Geometry check sheet. Reference: the model listing, model coordinates, mm. Face numbers are marked on the shaded views. A direction names the side the tool comes from. Round coordinates to 2 decimals unless told otherwise and drop trailing zeros. Order: outer loops, then holes, each group sorted by start corner. A loop starts at its lowest first (then second) coordinate and runs counter-clockwise, first axis right, second up.
(1) Sectioned sample at B-B (x = -46.05). Record the boundary of the cut face in (y, z), plus the area to 4 significant figures.
(2) Go/stop test with flat-tipped pins: pin 1 (7.5 mm diameter, centred on y = 10.5, z = -4.5, fed in from +X); pin 2 (15.5 mm diameter, centred on x = -6.5, z = 2.5, fed in from +Y); pin 3 (1 mm diameter, centred on x = 2, z = -17.5, fed in from -Y). Record where each tip stops, or that it passes through.
(3) Release check for a two-part mould opening along Z. For the marked faces 4, 5 and 6 record: +Z half, -Z half, draft (parallel to the pull), parting line (faces both ways), or undercut.
(4) Sectioned sample at C-C (z = 0). Give the number of separate pieces and of enclosed holes in the cut face, plus the area to 3 significant figures.
(5) Sectioned sample at A-A (y = 13.5). Record the boundary of the cut face in (x, z).
(6) Sectioned sample at D-D (x = -28.5). Record the boundary of the cut face in (y, z), plus the area to 3 significant figures.
(7) Set-up check for the marked faces 1, 2 and 3: record each of +Z, -Z, +X, -X, +Y, -Y from which the full face is reachable in a straight line by a thin tool's end or side.
(8) Material ranges on line 1 along Y through (x, z) = (7, 15); line 2 along X through (y, z) = (1.8, 20.9); line 3 along Z through (x, y) = (16, 1.5), recorded low to high.
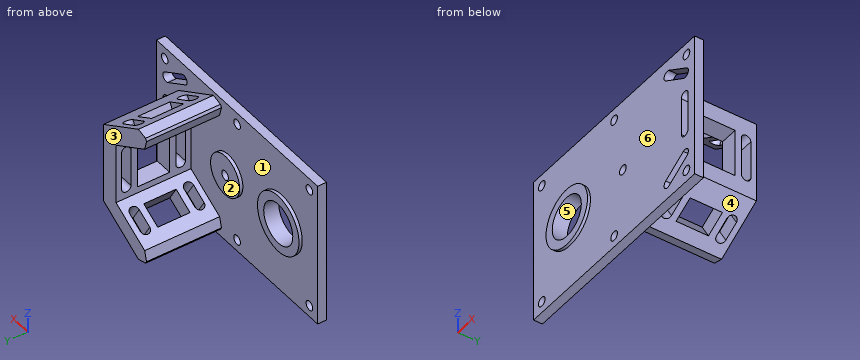
from build123d import *

# Parameters (mm, degrees)
SKETCH1_W            = 77.5936289
SKETCH1_H            = 49.9
SKETCH1_R            = 7
SKETCH1_R_2          = 1.6
BOSS_EXTRUDE6_DEPTH  = 3
SKETCH7_R            = 10
SKETCH7_R_2          = 7
BOSS_EXTRUDE7_DEPTH  = 1.1
BOSS_EXTRUDE9_START  = 1
SKETCH9_R            = 10
SKETCH9_R_2          = 7
BOSS_EXTRUDE9_DEPTH  = 1
SKETCH8_R            = 1.5
BOSS_EXTRUDE8_DEPTH  = 0.1
BOSS_EXTRUDE10_DEPTH = 25.5
SKETCH11_W           = 7.767839657
SKETCH11_H           = 11
CUT_EXTRUDE3_DEPTH   = 60.057720192
CUT_EXTRUDE4_DEPTH   = 11
CHAMFER2_SIZE        = 2.5
CHAMFER3_SIZE        = 2.5
SKETCH12_R           = 1.6
CUT_EXTRUDE5_DEPTH   = 4.2
SKETCH15_W           = 16.405303922
SKETCH15_H           = 11
CUT_EXTRUDE6_DEPTH   = 6
CUT_EXTRUDE7_DEPTH   = 3


with BuildPart() as part:
    # Sketch1 → Boss-Extrude6 (new body)
    with BuildSketch(Plane(origin=(0, 0, 0), x_dir=(1, 0, 0), z_dir=(0, 1, 0))):
        with Locations((-11.20318555, 0.05)):
            Rectangle(SKETCH1_W, SKETCH1_H)
        with Locations(Location((-32.593845483, 0, 0), (0, 0, 270))):
            Circle(SKETCH1_R, mode=Mode.SUBTRACT)
        with Locations(Location((-46.05, 21.05, 0), (0, 0, 270))):
            Circle(SKETCH1_R_2, mode=Mode.SUBTRACT)
        with Locations(Location((-46.05, -20.9, 0), (0, 0, 270))):
            Circle(SKETCH1_R_2, mode=Mode.SUBTRACT)
        with Locations(Location((23.6436289, -20.9, 0), (0, 0, 270))):
            Circle(SKETCH1_R_2, mode=Mode.SUBTRACT)
        with Locations(Location((23.6436289, 21.05, 0), (0, 0, 270))):
            Circle(SKETCH1_R_2, mode=Mode.SUBTRACT)
        with Locations(Location((-11.20318555, -20.9, 0), (0, 0, 270))):
            Circle(SKETCH1_R_2, mode=Mode.SUBTRACT)
        with Locations(Location((-11.20318555, 21.05, 0), (0, 0, 270))):
            Circle(SKETCH1_R_2, mode=Mode.SUBTRACT)
    extrude(amount=BOSS_EXTRUDE6_DEPTH)

    # Sketch7 → Boss-Extrude7 (add)
    # profile 1 of 2: a face of its own
    with BuildSketch(Plane(origin=(0, 3, 0), x_dir=(1, 0, 0), z_dir=(0, 1, 0))):
        with Locations(Location((-32.593845483, 0, 0), (0, 0, 90))):
            Circle(SKETCH7_R)
        with Locations(Location((-32.593845483, 0, 0), (0, 0, 270))):
            Circle(SKETCH7_R_2, mode=Mode.SUBTRACT)
    # profile 2 of 2: a face of its own
    with BuildSketch(Plane(origin=(0, 3, 0), x_dir=(1, 0, 0), z_dir=(0, 1, 0))):
        with Locations(Location((-6.993845483, 0, 0), (0, 0, 90))):
            Circle(SKETCH7_R_2)
    extrude(amount=BOSS_EXTRUDE7_DEPTH)

    # Sketch9 → Boss-Extrude9 (add)
    with BuildSketch(Plane.XZ.offset(BOSS_EXTRUDE9_START)):
        with Locations(Location((-32.593845483, 0, 0), (0, 0, 270))):
            Circle(SKETCH9_R)
        with Locations(Location((-32.593845483, 0, 0), (0, 0, 270))):
            Circle(SKETCH9_R_2, mode=Mode.SUBTRACT)
    extrude(amount=-BOSS_EXTRUDE9_DEPTH)

    # Sketch8 → Boss-Extrude8 (add)
    with BuildSketch(Plane(origin=(0, 4.1, 0), x_dir=(1, 0, 0), z_dir=(0, 1, 0))):
        with Locations(Location((-6.993845483, 0, 0), (0, 0, 270))):
            Circle(SKETCH8_R)
    extrude(amount=BOSS_EXTRUDE8_DEPTH)

    # Sketch10 → Boss-Extrude10 (add)
    with BuildSketch(Plane(origin=(0, 3, 0), x_dir=(1, 0, 0), z_dir=(0, 1, 0))):
        Polygon((11.006154517, 10.392304845), (-4.95090881, 19.605119652), (-1.95090881, 24.801272075), (17.006154517, 13.856406461), (17.006154517, -13.856406461), (-1.95090881, -24.801272075), (-4.95090881, -19.605119652), (11.006154517, -10.392304845), align=None)
    extrude(amount=BOSS_EXTRUDE10_DEPTH)

    # Sketch11 → Cut-Extrude3 (cut)
    with BuildSketch(Plane(origin=(10.251538629, 0, 17.756185762), x_dir=(0.8660254037844386, 0, -0.5000000000000001), z_dir=(0.5000000000000001, 0, 0.8660254037844386))):
        with BuildLine():
            Line((-6.090172627, 26.6), (-0.200441398, 26.6))
            ThreePointArc((-0.200441398, 26.6), (1.399558602, 25), (-0.200441398, 23.4))
            Line((-0.200441398, 23.4), (-6.090172627, 23.4))
            ThreePointArc((-6.090172627, 23.4), (-7.690172627, 25), (-6.090172627, 26.6))
        make_face()
        with BuildLine():
            Line((-6.090172627, 8.1), (-0.200441398, 8.1))
            ThreePointArc((-0.200441398, 8.1), (1.399558602, 6.5), (-0.200441398, 4.9))
            Line((-0.200441398, 4.9), (-6.090172627, 4.9))
            ThreePointArc((-6.090172627, 4.9), (-7.690172627, 6.5), (-6.090172627, 8.1))
        make_face()
        with Locations((-3.145307013, 15.75)):
            Rectangle(SKETCH11_W, SKETCH11_H)
    cut_extrude3 = extrude(amount=-CUT_EXTRUDE3_DEPTH, mode=Mode.SUBTRACT)

    # Mirror4: Cut-Extrude3 across plane
    add(cut_extrude3.mirror(Plane.XY), mode=Mode.SUBTRACT)

    # Sketch13 → Cut-Extrude4 (cut)
    with BuildSketch(Plane(origin=(0, 3, 0), x_dir=(1, 0, 0), z_dir=(0, 1, 0))):
        with BuildLine():
            Line((13.661155176, -18.122101509), (22.159879545, -13.215360707))
            ThreePointArc((22.159879545, -13.215360707), (24.352350318, -13.80283148), (23.764879545, -15.995302253))
            Line((23.764879545, -15.995302253), (15.266155176, -20.902043055))
            ThreePointArc((15.266155176, -20.902043055), (13.073684403, -20.314572282), (13.661155176, -18.122101509))
        make_face()
    cut_extrude4 = extrude(amount=-CUT_EXTRUDE4_DEPTH, mode=Mode.SUBTRACT)

    # Mirror5: Cut-Extrude4 across plane
    add(cut_extrude4.mirror(Plane.XY), mode=Mode.SUBTRACT)

    # Chamfer2
    chamfer2_edges = [part.edges().sort_by_distance(p)[0] for p in [
        (-4.95090881, 15.75, 19.605119652),
        (-4.95090881, 15.75, -19.605119652),
    ]]
    chamfer(chamfer2_edges, length=CHAMFER2_SIZE)

    # Chamfer3
    chamfer3_edges = [part.edges().sort_by_distance(p)[0] for p in [
        (-1.95090881, 15.75, 24.801272075),
        (-1.95090881, 15.75, -24.801272075),
    ]]
    chamfer(chamfer3_edges, length=CHAMFER3_SIZE)

    # Sketch12 → Cut-Extrude5 (cut)
    with BuildSketch(Plane(origin=(0, 4.2, 0), x_dir=(1, 0, 0), z_dir=(0, 1, 0))):
        with Locations(Location((-6.993845483, 0, 0), (0, 0, 270))):
            Circle(SKETCH12_R)
    extrude(amount=-CUT_EXTRUDE5_DEPTH, mode=Mode.SUBTRACT)

    # Sketch15 → Cut-Extrude6 (cut)
    with BuildSketch(Plane(origin=(17.006154517, 0, 0), x_dir=(0, 0, -1), z_dir=(1, 0, 0))):
        with Locations((0, 15.75)):
            Rectangle(SKETCH15_W, SKETCH15_H)
        with BuildLine():
            Line((-6.602651961, 26.6), (6.602651961, 26.6))
            ThreePointArc((6.602651961, 26.6), (8.202651961, 25), (6.602651961, 23.4))
            Line((6.602651961, 23.4), (-6.602651961, 23.4))
            ThreePointArc((-6.602651961, 23.4), (-8.202651961, 25), (-6.602651961, 26.6))
        make_face()
        with BuildLine():
            Line((-6.602651961, 4.9), (6.602651961, 4.9))
            ThreePointArc((6.602651961, 4.9), (8.202651961, 6.5), (6.602651961, 8.1))
            Line((6.602651961, 8.1), (-6.602651961, 8.1))
            ThreePointArc((-6.602651961, 8.1), (-8.202651961, 6.5), (-6.602651961, 4.9))
        make_face()
    extrude(amount=-CUT_EXTRUDE6_DEPTH, mode=Mode.SUBTRACT)

    # Sketch16 → Cut-Extrude7 (cut)
    with BuildSketch(Plane(origin=(0, 3, 0), x_dir=(1, 0, 0), z_dir=(0, 1, 0))):
        with BuildLine():
            Line((21.215137645, -6.479589384), (21.215137645, 6.479589384))
            ThreePointArc((21.215137645, 6.479589384), (22.820137645, 8.084589384), (24.425137645, 6.479589384))
            Line((24.425137645, 6.479589384), (24.425137645, -6.479589384))
            ThreePointArc((24.425137645, -6.479589384), (22.820137645, -8.084589384), (21.215137645, -6.479589384))
        make_face()
    extrude(amount=-CUT_EXTRUDE7_DEPTH, mode=Mode.SUBTRACT)


solid = part.part
Answer below:
1. outline: (0, -25) - (3, -25) - (3, -22.65) - (0, -22.65) - close; (0, -19.45) - (3, -19.45) - (3, 19.3) - (0, 19.3) - close; (0, 22.5) - (3, 22.5) - (3, 24.9) - (0, 24.9) - close
1. area: 130.5 mm2
2. pin 1: stops at x = 17.01
2. pin 2: stops at y = 4.1
2. pin 3: stops at y = 0
3. face 4: -Z half
3. face 5: undercut
3. face 6: draft
4. separate pieces: 7
4. enclosed holes: 0
4. area: 245 mm2
5. outline: (-3.7, -21.77) - (-3.2, -22.64) - (0.21, -23.55) - (4.16, -21.27) - (1.16, -16.07) - (-2.79, -18.36) - close; (-3.7, 21.77) - (-2.79, 18.36) - (1.16, 16.07) - (4.16, 21.27) - (0.21, 23.55) - (-3.2, 22.64) - close; (7.89, -12.19) - (10.89, -17.39) - (17.01, -13.86) - (17.01, -8.2) - (11.01, -8.2) - (11.01, -10.39) - close; (7.89, 12.19) - (11.01, 10.39) - (11.01, 8.2) - (17.01, 8.2) - (17.01, 13.86) - (10.89, 17.39) - close
6. outline: (-1, -9.12) - (0, -9.12) - (0, -25) - (3, -25) - (3, -9.12) - (4.1, -9.12) - (4.1, -5.68) - (-1, -5.68) - close; (-1, 5.68) - (4.1, 5.68) - (4.1, 9.12) - (3, 9.12) - (3, 24.9) - (0, 24.9) - (0, 9.12) - (-1, 9.12) - close
6. area: 130 mm2
7. face 1: +Y
7. face 2: -X, +Y
7. face 3: +Z, -Z, +X, -X, +Y
8. line 1: y = 0 to 4.9, 8.1 to 10.25, 21.25 to 23.4, 26.6 to 28.5
8. line 2: x = -50 to -47.65, -44.45 to -12.8, -9.6 to 13.66, 15.27 to 22.04, 25.24 to 27.59
8. line 3: z = -25 to -20.48, -16.77 to 16.77, 20.48 to 24.9
